Could you check a few things on this model? Use its own coordinates, in mm. Face numbers are marked on the shaded views. A direction names the side the tool comes from. Round coordinates to 2 decimals unless told otherwise and drop trailing zeros. Loops run counter-clockwise (first coordinate to the right, second up) from the corner with the lowest first, then second, coordinate; pieces in that order, holes last. Notation, with made-up numbers: (-22.5, -20) -> (18.5, -20) arc R8 cw to (18.5, -15) -> close; hole circle Ø10 at (-10, 63). An arc over 180 degrees is marked (long way). Write each question's results on one line, items separated by ' | '.
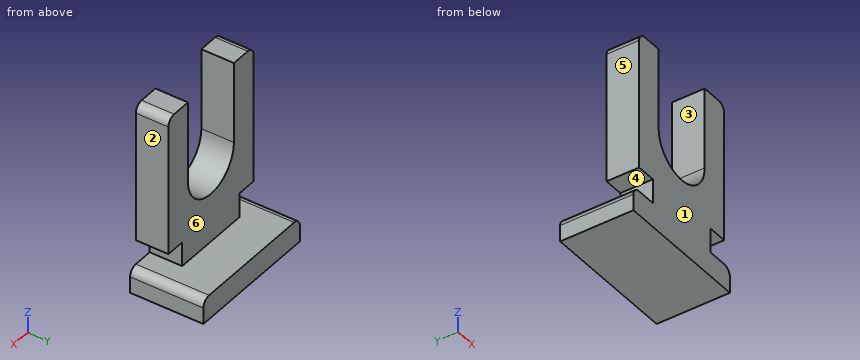
from build123d import *

# Parameters (mm, degrees)
ESQUISSE1_W        = 84
ESQUISSE1_H        = 45
BOSS_EXTRU_1_DEPTH = 15
BOSS_EXTRU_2_DEPTH = 20
CONG_1_R           = 5


with BuildPart() as part:
    # Esquisse1 → Boss.-Extru.1 (new body)
    with BuildSketch(Plane.XY):
        Rectangle(ESQUISSE1_W, ESQUISSE1_H)
    extrude(amount=BOSS_EXTRU_1_DEPTH)

    # Esquisse2 → Boss.-Extru.2 (add)
    with BuildSketch(Plane.XZ.offset(22.5)):
        with BuildLine():
            Line((37, 115), (37, 30))
            Line((37, 30), (25, 30))
            Line((25, 30), (25, 15))
            Line((25, 15), (0, 15))
            Line((0, 15), (-25, 15))
            Line((-25, 15), (-25, 30))
            Line((-25, 30), (-37, 30))
            Line((-37, 30), (-37, 115))
            Line((-37, 115), (-20, 115))
            Line((-20, 115), (-20, 65))
            ThreePointArc((-20, 65), (0, 45), (20, 65))
            Line((20, 65), (20, 115))
            Line((20, 115), (37, 115))
        make_face()
    extrude(amount=-BOSS_EXTRU_2_DEPTH)

    # Congé1
    cong_1_edges = [part.edges().sort_by_distance(p)[0] for p in [
        (42, 0, 15),
        (37, -12.5, 115),
        (-37, -12.5, 115),
        (-42, 0, 15),
    ]]
    fillet(cong_1_edges, radius=CONG_1_R)


solid = part.part
1) I want a section at D-D, the plane x = 0. Write out the boundary of the cut face in (y, z), plus the area to 4 significant figures.
Model answer:
outline: (-22.5, 0) -> (22.5, 0) -> (22.5, 15) -> (-2.5, 15) -> (-2.5, 45) -> (-22.5, 45) -> close | area: 1,275 mm2
2) I'm going to push flat-ended pins straight in: pin 1 (10 mm diameter, centred on y = -12.5, z = 59.5, fed in from -X); pin 2 (16.5 mm diameter, centred on y = -14, z = 22, fed in from -X); pin 3 (13.5 mm diameter, centred on x = -5, y = -11, fed in from +Z); pin 4 (9.5 mm diameter, centred on x = 32, y = -11.5, fed in from -Z). Where does each tip first touch, or does it pass through?
Model answer:
pin 1: stops at x = -37 | pin 2: stops at x = -40.31 | pin 3: stops at z = 48.82 | pin 4: stops at z = 0
3) I want a section at A-A, the plane x = 30. Write out the boundary of the cut face in (y, z), plus the area to 4 significant figures.
Model answer:
outline: (-22.5, 0) -> (22.5, 0) -> (22.5, 15) -> (-22.5, 15) -> close; (-22.5, 30) -> (-2.5, 30) -> (-2.5, 115) -> (-22.5, 115) -> close | area: 2,375 mm2
4) I need wall thicknesses on line 1 (X direction, y = -11.5, z = 82); line 2 (Y direction, x = 27, z = 85.5); line 3 (Z direction, x = 21.5, y = 14). Which ranges of each line are inside material? Lowest first, please.
Model answer:
line 1: x = -37 to -20, 20 to 37 | line 2: y = -22.5 to -2.5 | line 3: z = 0 to 15
5) I want a section at B-B, the plane z = 69. Write out the boundary of the cut face in (x, y), plus the area to 3 significant figures.
Model answer:
outline: (-37, -22.5) -> (-20, -22.5) -> (-20, -2.5) -> (-37, -2.5) -> close; (20, -22.5) -> (37, -22.5) -> (37, -2.5) -> (20, -2.5) -> close | area: 680 mm2
6) I want a section at C-C, the plane y = 15.5. Write out the boundary of the cut face in (x, z), plus the area to 3 significant figures.
Model answer:
outline: (-42, 0) -> (42, 0) -> (42, 10) arc R5 ccw to (37, 15) -> (-37, 15) arc R5 ccw to (-42, 10) -> close | area: 1,250 mm2
7) For the marked faces 4, 5 and 6, which set-ups out of +Z, -Z, +X, -X, +Y, -Y let a thin tool reach every point of the face, with its end or its side?
Model answer:
face 4: -X, +Y, -Y | face 5: +Z, -X, +Y, -Y | face 6: +Z, +X, -X, +Y
8) If we mould it in two halves opening along X, with no side actions, what happens to the marked faces 1, 2 and 3? For each: released by +X, released by -X, zero draft, split by the parting line, or undercut.
Model answer:
face 1: zero draft | face 2: released by +X | face 3: undercut
